The model under review builds one solid part; all positions refer to its coordinate system, in mm. A direction names the side the tool comes from. Round coordinates to 2 decimals unless told otherwise and drop trailing zeros. Write each loop counter-clockwise with the first axis right and the second up, starting at its lowest first coordinate (ties: lowest second). Pieces come first, ordered by that corner, then holes. Notation, with made-up numbers: (46, 7) -> (103, 7) arc R31 ccw to (103, 33) -> close; hole circle Ø11 at (7, 39). An arc over 180 degrees is marked (long way). Return JSON: item names as keys, results as strings. Group by question number.
1. Take a section at D-D, the plane x = -19.05. Write out the cut boundary in (y, z) (3 decimals).
2. Take a section at B-B, the plane x = -6.35. Write out the cut boundary in (y, z) (3 decimals).
3. Take a section at A-A, the plane y = 19.05. Write out the cut boundary in (x, z) (3 decimals), then the cut area to 3 significant figures.
4. Mouldability with a two-part tool opening along Z and no side actions: class faces 3 (the flat face through (0, 2, -8)), 4 (the cylindrical face through (-22.03, 1.57, -10.46)), 5 (the flat face through (-13, 14, -3.175)) as pulls with the +Z half, pulls with the -Z half, needs draft (parallel to the pull), parting line crosses it, or undercut.
5. Clearance check with a flat-ended pin moving along its axis: P1, Ø11, axis at x = -7.5, z = -16.5, coming from the +Y side (3 decimals). State where the tip first meets the part, or that it passes through.
6. Take a section at C-C, the plane z = -19.05. Write out the cut boundary in (x, y) (3 decimals).
7. Tool access review of faces 1 (the flat face through (-13, 25.4, -2)), 2 (the flat face through (-13, 3.175, -14)): name each direction out of +Z, -Z, +X, -X, +Y, -Y from which nothing blocks a thin tool from reaching the whole face with its end or side.
8. For line 1 along Y through (x, z) = (-19.05, -2.3) (3 decimals); line 2 along Y through (x, z) = (-6.35, -1.05); line 3 along Z through (x, y) = (-19.5, 14) (3 decimals), list the stretches that pass through material, from the lowest coordinate up. Write a range as from..to.
Autodesk Inventor part; units mm, degrees
ref_plane "YZ Plane" through (0, 0, 0) normal (1, 0, 0) x (0, 1, 0)
ref_plane "XZ Plane" through (0, 0, 0) normal (0, 1, 0) x (-1, 0, 0)
ref_plane "XY Plane" through (0, 0, 0) normal (0, 0, 1) x (1, 0, 0)
sketch "Sketch1" plane through (0, 0, 0) normal (0, 1, 0) x (-1, 0, 0)
  line L0 (0, 0) -> (25.4, 0)
  line L1 (25.4, 0) -> (25.4, -25.4)
  line L2 (25.4, -25.4) -> (0, -25.4)
  line L3 (0, -25.4) -> (0, 0)
  circle A0 centre (6.35, -19.05) radius 3.175
  circle A1 centre (19.05, -9.525) radius 3.124
  line L4 (25.4, 0) -> (0, 0)
  line L5 (0, 0) -> (0, -3.175)
  line L6 (0, -3.175) -> (25.4, -3.175)
  line L7 (25.4, -3.175) -> (25.4, 0)
  dimension "d0" = 25.4
  dimension "d1" = 25.4
  dimension "d2" = 6.35
  dimension "d3" = 6.35
  dimension "d4" = 6.35
  dimension "d5" = 9.525
  dimension "d6" = 6.35
  dimension "d7" = 3.175
extrude "Extrusion1" add sketch "Sketch1" along normal blind 3.175 contours L6 L1 L2 L3
extrude "Extrusion2" add sketch "Sketch1" along normal blind 25.4 contours L0 L1 L6 L3
sketch "Sketch2" plane through (-25.4, 0, 0) normal (0, 0, 1) x (1, 0, 0)
  circle A0 centre (6.35, 19.05) radius 3.175
  line L0 (0, 25.4) -> (25.4, 25.4)
  line L1 (0, 0) -> (0, 25.4)
  circle A1 centre (19.05, 9.525) radius 3.175
  line L2 (25.4, 0) -> (25.4, 25.4)
  line L3 (0, 0) -> (25.4, 0)
  dimension "d12" = 6.35
  dimension "d13" = 6.35
  dimension "d14" = 6.35
  dimension "d15" = 6.35
  dimension "d16" = 9.525
  dimension "d17" = 6.35
extrude "Extrusion3" cut sketch "Sketch2" against normal through all contours A0 | A1
properties part number "connector1by1"
Output:
{
 "1": {"outline": "(0, -25.4) -> (3.175, -25.4) -> (3.175, -12.649) -> (0, -12.649) -> close; (0, -6.401) -> (3.175, -6.401) -> (3.175, -3.175) -> (15.875, -3.175) -> (15.875, 0) -> (0, 0) -> close; (22.225, -3.175) -> (25.4, -3.175) -> (25.4, 0) -> (22.225, 0) -> close"},
 "2": {"outline": "(0, -25.4) -> (3.175, -25.4) -> (3.175, -22.225) -> (0, -22.225) -> close; (0, -15.875) -> (3.175, -15.875) -> (3.175, -3.175) -> (6.35, -3.175) -> (6.35, 0) -> (0, 0) -> close; (12.7, -3.175) -> (25.4, -3.175) -> (25.4, 0) -> (12.7, 0) -> close"},
 "3": {"outline": "(-25.4, -3.175) -> (-22.225, -3.175) -> (-22.225, 0) -> (-25.4, 0) -> close; (-15.875, -3.175) -> (0, -3.175) -> (0, 0) -> (-15.875, 0) -> close", "area": "60.5 mm^2"},
 "4": {"face 3": "needs draft", "face 4": "undercut", "face 5": "pulls with the -Z half"},
 "5": {"P1": "stops at y = 3.175"},
 "6": {"outline": "(-25.4, 0) -> (-9.525, 0) -> (-9.525, 3.175) -> (-25.4, 3.175) -> close; (-3.175, 0) -> (0, 0) -> (0, 3.175) -> (-3.175, 3.175) -> close"},
 "7": {"face 1": "+Z, -Z, +X, -X, +Y", "face 2": "-Z, +X, -X, +Y"},
 "8": {"line 1": "y = 0..15.875, 22.225..25.4", "line 2": "y = 0..6.35, 12.7..25.4", "line 3": "z = -3.175..0"}
}
